from build123d import *

# Parameters (mm, degrees)
F1_DEPTH  = 12.7
F2_DEPTH  = 12.7
F3_R      = 10.2599361316
F4_DEPTH  = 127
F5_DEPTH  = 25.4
F6_DEPTH  = 12.7
F7_DEPTH  = 2.54
F8_DEPTH  = 25.4
F9_DEPTH  = 25.4
F10_DEPTH = 5.08


with BuildPart() as f1:
    # F0 (on Front) → F1 (new body)
    with BuildSketch(Plane.XZ):
        Polygon((28.0411653221, -5.1526171155), (28.0411653221, 20.8860766143), (16.4345689118, 20.8860766143), (-16.3516514003, 20.8860766143), (-27.6816412807, 20.8860766143), (-27.6816412807, -5.1526171155), align=None)
        Polygon((16.4345689118, 20.8860766143), (28.0411653221, 20.8860766143), (36.4657826722, 27.4914167821), (42.8281202912, 10.9493397176), (91.7288586497, 81.2863186002), (43.9798757434, 34.9366031587), (42.0971289277, 52.180416882), align=None)
        Polygon((-27.6816412807, 20.8860766143), (-16.3516514003, 20.8860766143), (-42.1405397356, 52.1064698696), (-43.9977906644, 34.9366031587), (-91.8636098504, 81.2863186002), (-42.8677536547, 10.9493397176), (-36.362465471, 27.4914167821), align=None)
    extrude(amount=F1_DEPTH)

    # F2 (add): a face of the model
    f2_faces = [f1.faces().sort_by_distance(p)[0] for p in [
        (26.0119318683, 0, 7.8667297494),
    ]]
    extrude(f2_faces, amount=F2_DEPTH)

    # F3 (on face) → F4 (join)
    with BuildSketch(Plane(origin=(0, 0, -5.1526171155), x_dir=(1, 0, 0), z_dir=(0, 0, -1))):
        Circle(F3_R)
    extrude(amount=F4_DEPTH)

    # F5 (cut): a face of the model
    f5_faces = [f1.faces().sort_by_distance(p)[0] for p in [
        (0, 0, -132.1526171155),
    ]]
    extrude(f5_faces, amount=-F5_DEPTH, mode=Mode.SUBTRACT)

    # F6 (add): a face of the model
    f6_faces = [f1.faces().sort_by_distance(p)[0] for p in [
        (0, 0, -106.7526171155),
    ]]
    extrude(f6_faces, amount=F6_DEPTH)

    # F7 (cut): a face of the model
    f7_faces = [f1.faces().sort_by_distance(p)[0] for p in [
        (0, 0, -119.4526171155),
    ]]
    extrude(f7_faces, amount=-F7_DEPTH, mode=Mode.SUBTRACT)

    # F8 (cut): a face of the model
    f8_faces = [f1.faces().sort_by_distance(p)[0] for p in [
        (26.0119318683, -12.7, 7.8667297494),
    ]]
    extrude(f8_faces, amount=-F8_DEPTH, mode=Mode.SUBTRACT)

    # F9 (add): a face of the model
    f9_faces = [f1.faces().sort_by_distance(p)[0] for p in [
        (0, 0, -5.1526171155),
    ]]
    extrude(f9_faces, amount=F9_DEPTH)

    # F10 (cut): a face of the model
    f10_faces = [f1.faces().sort_by_distance(p)[0] for p in [
        (0, 0, 20.2473828845),
    ]]
    extrude(f10_faces, amount=-F10_DEPTH, mode=Mode.SUBTRACT)


solid = f1.part
For this review, take the finished solid that the model builds, in its own axes (mm). Coordinates: 2 decimals unless noted, no trailing zeros. Write each loop counter-clockwise with the first axis right and the second up, starting at its lowest first coordinate (ties: lowest second). Pieces come first, ordered by that corner, then holes. Notation, with made-up numbers: (3, 89) -> (37, 89) arc R21 cw to (37, 117) -> close; hole circle Ø11 at (68.5, -39). An arc over 180 degrees is marked (long way). Write each question's results on one line, items separated by ' | '. Start each with the question number.
1) Wall thickness on L1, parallel to Y at x = -0.5, z = -80.5; L2, parallel to X at y = -4.25, z = -5: over which ranges is each line inside the solid? List them lowest first. Write a range as [from, to].
2) Consider section C-C (z = -83). Write out the cut boundary in (x, y).
3) Insertion check: pin 1 (2 mm diameter, centred on x = -4, z = -101, fed in from +Y); pin 2 (10 mm diameter, centred on y = -6, z = -77.5, fed in from +X); pin 3 (8 mm diameter, centred on y = -5, z = 0, fed in from -X). Each pin has a flat end and moves straight along its axis. Give the tip position at first contact, or say it passes through.
4) Consider section B-B (y = 5). Write out the cut boundary in (x, z), plus the area to 3 significant figures.
5) Consider section A-A (x = 7.25). Write out the cut boundary in (y, z).
Geometry says:
1) L1: [-10.25, 10.25] | L2: [-9.34, 9.34]
2) outline: circle Ø20.52 at (0, 0)
3) pin 1: y = 9.81 | pin 2: x = 10.21 | pin 3: x = -10.21
4) outline: (-8.96, -116.91) -> (8.96, -116.91) -> (8.96, 15.17) -> (-8.96, 15.17) -> close | area: 2,370 mm^2
5) outline: (-7.26, -116.91) -> (7.26, -116.91) -> (7.26, 15.17) -> (-7.26, 15.17) -> close
